```python
from build123d import *

# Parameters (mm, degrees)
SKETCH_1_W          = 41
SKETCH_1_H          = 30
EXTRUDE_1_DEPTH     = 10
SKETCH_3_W          = 30
SKETCH_3_H          = 10
CUT_EXTRUDE_2_DEPTH = 3
EXTRUDE_3_DEPTH     = 30
SKETCH_6_W          = 20
SKETCH_6_H          = 30
CUT_EXTRUDE_5_DEPTH = 9
SKETCH_2_R          = 1.1
CUT_EXTRUDE_1_DEPTH = 15
SKETCH_8_R          = 1.5
CUT_EXTRUDE_6_DEPTH = 52.594573358
SKETCH_4_R          = 1.1
CUT_EXTRUDE_3_DEPTH = 10
CUT_EXTRUDE_7_DEPTH = 54.572380944
CUT_EXTRUDE_8_DEPTH = 4
SKETCH_11_W         = 4.132049734
SKETCH_11_H         = 3.255839909
CUT_EXTRUDE_9_DEPTH = 54.572380944


with BuildPart() as part:
    # Эскиз1 → Бобышка-Вытянуть1 (new body)
    with BuildSketch(Plane(origin=(0, 0, 0), x_dir=(1, 0, 0), z_dir=(0, 1, 0))):
        with Locations((20.5, 15)):
            Rectangle(SKETCH_1_W, SKETCH_1_H)
    extrude(amount=EXTRUDE_1_DEPTH)

    # Эскиз3 → Вырез-Вытянуть2 (cut)
    with BuildSketch(Plane.ZY):
        with Locations((-15, 5)):
            Rectangle(SKETCH_3_W, SKETCH_3_H)
    extrude(amount=-CUT_EXTRUDE_2_DEPTH, mode=Mode.SUBTRACT)

    # Эскиз7 → Бобышка-Вытянуть3 (add)
    with BuildSketch(Plane(origin=(0, 0, -30), x_dir=(-1, 0, 0), z_dir=(0, 0, -1))):
        Polygon((-39, 17), (-21, 17), (-9, 10), (-39, 10), align=None)
    extrude(amount=-EXTRUDE_3_DEPTH)

    # Эскиз6 → Вырез-Вытянуть5 (cut)
    with BuildSketch(Plane.XZ):
        with Locations((31, -15)):
            Rectangle(SKETCH_6_W, SKETCH_6_H)
    extrude(amount=-CUT_EXTRUDE_5_DEPTH, mode=Mode.SUBTRACT)

    # Эскиз2 → Вырез-Вытянуть1 (cut)
    with BuildSketch(Plane(origin=(39, 0, 0), x_dir=(0, 0, -1), z_dir=(1, 0, 0))):
        with Locations((4, 12.5)):
            Circle(SKETCH_2_R)
        with Locations((26, 12.5)):
            Circle(SKETCH_2_R)
    extrude(amount=-CUT_EXTRUDE_1_DEPTH, mode=Mode.SUBTRACT)

    # Эскиз8 → Вырез-Вытянуть6 (cut, through all)
    with BuildSketch(Plane(origin=(0, 9, 0), x_dir=(1, 0, 0), z_dir=(0, 1, 0))):
        with Locations(Location((35.949747468, 19.949747468, 0), (0, 0, 270))):
            Circle(SKETCH_8_R)
        with Locations(Location((35.949747468, 10.050252532, 0), (0, 0, 270))):
            Circle(SKETCH_8_R)
        with Locations(Location((26.050252532, 10.050252532, 0), (0, 0, 270))):
            Circle(SKETCH_8_R)
        with Locations(Location((26.050252532, 19.949747468, 0), (0, 0, 270))):
            Circle(SKETCH_8_R)
    extrude(amount=CUT_EXTRUDE_6_DEPTH, mode=Mode.SUBTRACT)

    # Эскиз4 → Вырез-Вытянуть3 (cut)
    with BuildSketch(Plane.ZY.offset(-3)):
        with Locations((-20, 5.4)):
            Circle(SKETCH_4_R)
        with Locations((-10, 5.4)):
            Circle(SKETCH_4_R)
    extrude(amount=-CUT_EXTRUDE_3_DEPTH, mode=Mode.SUBTRACT)

    # Эскиз9 → Вырез-Вытянуть7 (cut, through all)
    with BuildSketch(Plane(origin=(0, 0, -30), x_dir=(-1, 0, 0), z_dir=(0, 0, -1))):
        Polygon((-21, 9), (-21, 0), (-11, 0), align=None)
    extrude(amount=-CUT_EXTRUDE_7_DEPTH, mode=Mode.SUBTRACT)

    # Эскиз10 → Вырез-Вытянуть8 (cut)
    with BuildSketch(Plane(origin=(0, 17, 0), x_dir=(1, 0, 0), z_dir=(0, 1, 0))):
        Polygon((26.050252532, 23.240644003), (23.200252532, 21.595195735), (23.200252532, 18.304299201), (26.050252532, 16.658850934), (28.900252532, 18.304299201), (28.900252532, 21.595195735), align=None)
        Polygon((35.949747468, 23.240644003), (33.099747468, 21.595195735), (33.099747468, 18.304299201), (35.949747468, 16.658850934), (38.799747468, 18.304299201), (38.799747468, 21.595195735), align=None)
        Polygon((35.949747468, 13.341149066), (33.099747468, 11.695700799), (33.099747468, 8.404804265), (35.949747468, 6.759355997), (38.799747468, 8.404804265), (38.799747468, 11.695700799), align=None)
        Polygon((26.050252532, 13.341149066), (23.200252532, 11.695700799), (23.200252532, 8.404804265), (26.050252532, 6.759355997), (28.900252532, 8.404804265), (28.900252532, 11.695700799), align=None)
    extrude(amount=-CUT_EXTRUDE_8_DEPTH, mode=Mode.SUBTRACT)

    # Эскиз11 → Вырез-Вытянуть9 (cut, through all)
    with BuildSketch(Plane(origin=(0, 0, -30), x_dir=(-1, 0, 0), z_dir=(0, 0, -1))):
        with Locations((-41.066024867, 8.372080046)):
            Rectangle(SKETCH_11_W, SKETCH_11_H)
    extrude(amount=-CUT_EXTRUDE_9_DEPTH, mode=Mode.SUBTRACT)


solid = part.part
```
Input: part model. Units: mm. Frame: model coordinates. A direction names the side the tool comes from. Round coordinates to 2 decimals unless told otherwise and drop trailing zeros. Order: outer loops, then holes, each group sorted by start corner. A loop starts at its lowest first (then second) coordinate and runs counter-clockwise, first axis right, second up. Notation, with made-up numbers: (-37.75, -5.5) - (-6.75, -5.5) arc R21 cw to (-6.75, 31.5) - close; hole circle Ø4 at (50, 16). An arc over 180 degrees is marked (long way). Answer in a Markdown table with one row per item.
Item 1: Pin query (flat end, axial travel): pin 1 (1.7 mm diameter, centred on x = 25.5, z = -19, fed in from +Y); pin 2 (1.1 mm diameter, centred on y = 6, z = -20.5, fed in from -X); pin 3 (1.8 mm diameter, centred on y = 12.5, z = -4, fed in from -X); pin 4 (2 mm diameter, centred on y = 3.5, z = -7, fed in from +X). Return the tip coordinate at first contact, or that it passes through.
Model answer:
| item | result |
|---|---|
| pin 1 | stops at y = 13 |
| pin 2 | stops at x = 3 |
| pin 3 | stops at x = 11.74 |
| pin 4 | stops at x = 16 |
Item 2: Section query C-C (y = 12.5). Return the cut outline in (x, z).
Model answer:
| item | result |
|---|---|
| outline | (13.29, -30) - (39, -30) - (39, -27.1) - (24, -27.1) - (24, -24.9) - (39, -24.9) - (39, -5.1) - (24, -5.1) - (24, -2.9) - (39, -2.9) - (39, 0) - (13.29, 0) - close; hole circle Ø3 at (26.05, -19.95); hole circle Ø3 at (26.05, -10.05); hole circle Ø3 at (35.95, -19.95); hole circle Ø3 at (35.95, -10.05) |
Item 3: Section query A-A (z = -20). Return the cut outline in (x, y), then the cut area to 3 significant figures.
Model answer:
| item | result |
|---|---|
| outline | (3, 0) - (11, 0) - (21, 9) - (24.55, 9) - (24.55, 13) - (23.2, 13) - (23.2, 17) - (21, 17) - (9, 10) - (3, 10) - (3, 6.5) - (13, 6.5) - (13, 4.3) - (3, 4.3) - close; (27.55, 9) - (34.45, 9) - (34.45, 13) - (33.1, 13) - (33.1, 17) - (28.9, 17) - (28.9, 13) - (27.55, 13) - close; (37.45, 9) - (39, 9) - (39, 17) - (38.8, 17) - (38.8, 13) - (37.45, 13) - close |
| area | 229 mm² |
Item 4: Section query B-B (x = 30.5). Return the cut outline in (y, z).
Model answer:
| item | result |
|---|---|
| outline | (9, -30) - (17, -30) - (17, 0) - (9, 0) - close; hole circle Ø2.2 at (12.5, -26); hole circle Ø2.2 at (12.5, -4) |
Item 5: Section query D-D (z = -4). Return the cut outline in (x, y).
Model answer:
| item | result |
|---|---|
| outline | (3, 0) - (11, 0) - (21, 9) - (39, 9) - (39, 11.4) - (24, 11.4) - (24, 13.6) - (39, 13.6) - (39, 17) - (21, 17) - (9, 10) - (3, 10) - close |
Item 6: Line query: line 1 (Z direction, x = 8, y = 5.25); line 2 (Y direction, x = 5, z = -20); line 3 (X direction, y = 14.5, z = -18.5). Output: solid intervals per line, ascending.
Model answer:
| item | result |
|---|---|
| line 1 | z = -30 to -21.09, -18.91 to -11.09, -8.91 to 0 |
| line 2 | y = 0 to 4.3, 6.5 to 10 |
| line 3 | x = 16.71 to 23.2, 28.9 to 33.1, 38.8 to 39 |
Item 7: Reachability of faces 3 (the flat face through (37.355, 15.028, -17.47)), 4 (the cylindrical face through (36.4, 10.97, -18.52)), 5 (the cylindrical face through (31.6, 11.83, -25.13)) from +Z, -Z, +X, -X, +Y, -Y: full face, straight path, thin tool, end or side. Return the list, or none.
Model answer:
| item | result |
|---|---|
| face 3 | +Y |
| face 4 | +Y, -Y |
| face 5 | +X |
Item 8: Mould query, pull axis Z, two halves, no side actions, for faces 1 (the flat face through (27.495, 15.028, -12.507)), 2 (the flat face through (30, 9, -15)). Classes: released by +Z, released by -Z, zero draft, split by the parting line, or undercut.
Model answer:
| item | result |
|---|---|
| face 1 | undercut |
| face 2 | zero draft |
